The drawing under review shows one solid part. Ordinate dimensions are in mm from its lowest x, y, z. Round coordinates to 2 decimals unless told otherwise and drop trailing zeros. Write each loop counter-clockwise with the first axis right and the second up, starting at its lowest first coordinate (ties: lowest second). Pieces come first, ordered by that corner, then holes. Notation, with made-up numbers: (50.5, 43) -> (64.5, 43) arc R20 cw to (64.5, 65) -> close; hole circle Ø8 at (16.5, -20.5). An arc over 180 degrees is marked (long way). Use CSV: the item, a comma, the result in double quotes. Start each with the question number.
1) Take a section at D-D, the plane z = 1.5. Give the boundary of the cut face in (x, y), then the cut area to 3 significant figures.
2) Wall thickness on probe 1 along X at (y, z) = (19.8, 1.2) (1 decimal); probe 2 along Z at (x, y) = (33.5, 18.5); probe 3 along Y at (x, z) = (21, 1.25): over which ranges is each line inside the solid? List them lowest first. Write a range as [from, to].
3) Take a section at B-B, the plane z = 5.5. Give the boundary of the cut face in (x, y).
4) For pin 1 Ø4 at (x, y) = (9.5, 19.8) entering from -Z; pin 2 Ø4 at (x, y) = (32.75, 6.38) entering from +Z, all flat-tipped, find the tip position at first contact; note any pin that passes through.
5) Take a section at A-A, the plane x = 25. Give the boundary of the cut face in (y, z).
6) Mouldability with a two-part tool opening along X and no side actions: class the marked faces 1, 2 and 3 as released by +X, released by -X, zero draft, split by the parting line, or undercut.
7) Take a section at C-C, the plane y = 19.8. Give the boundary of the cut face in (x, z).
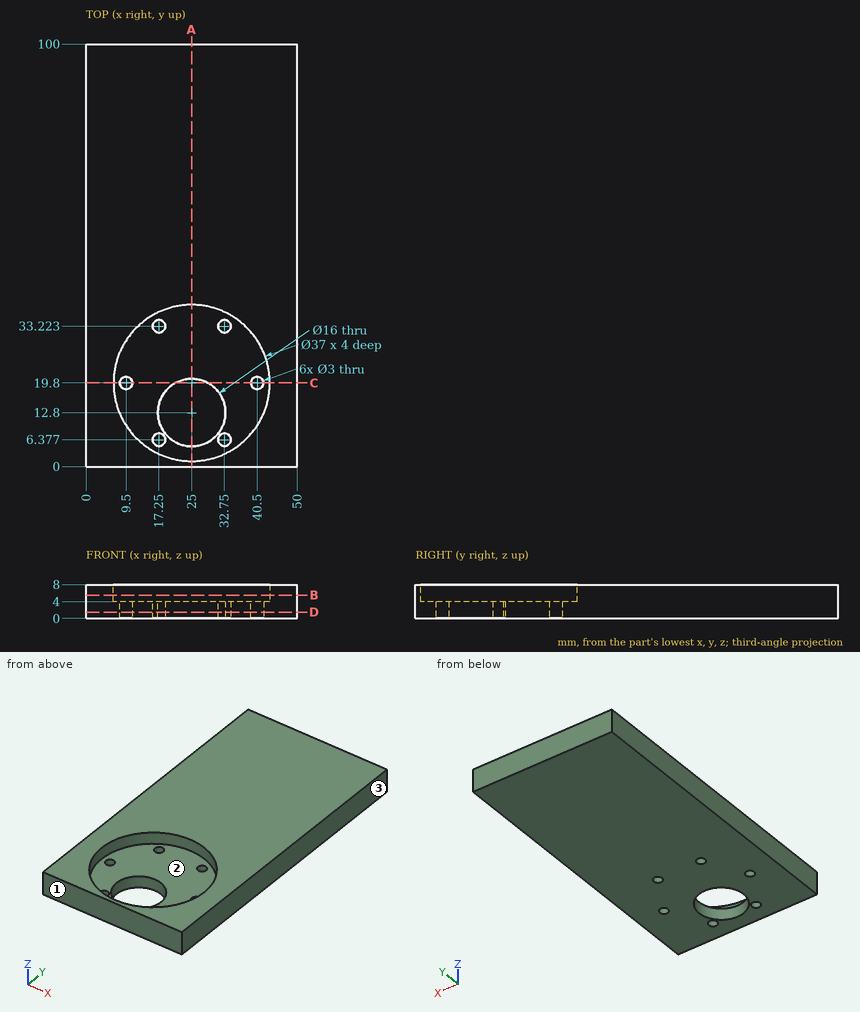
Values found:
1,outline,"(0, 0) -> (50, 0) -> (50, 100) -> (0, 100) -> close; hole circle Ø3 at (9.5, 19.8); hole circle Ø3 at (17.25, 6.38); hole circle Ø3 at (17.25, 33.22); hole circle Ø16 at (25, 12.8); hole circle Ø3 at (32.75, 6.38); hole circle Ø3 at (32.75, 33.22); hole circle Ø3 at (40.5, 19.8)"
1,area,"4,760 mm²"
2,probe 1,"[0, 8], [11, 21.1], [28.9, 39], [42, 50]"
2,probe 2,"[0, 4]"
2,probe 3,"[0, 5.87], [19.73, 100]"
3,outline,"(0, 0) -> (50, 0) -> (50, 100) -> (0, 100) -> close; hole circle Ø37 at (25, 19.8)"
4,pin 1,"z = 0"
4,pin 2,"z = 4"
5,outline,"(0, 0) -> (4.8, 0) -> (4.8, 4) -> (1.3, 4) -> (1.3, 8) -> (0, 8) -> close; (20.8, 0) -> (100, 0) -> (100, 8) -> (38.3, 8) -> (38.3, 4) -> (20.8, 4) -> close"
6,face 1,"zero draft"
6,face 2,"undercut"
6,face 3,"released by +X"
7,outline,"(0, 0) -> (8, 0) -> (8, 4) -> (6.5, 4) -> (6.5, 8) -> (0, 8) -> close; (11, 0) -> (21.13, 0) -> (21.13, 4) -> (11, 4) -> close; (28.87, 0) -> (39, 0) -> (39, 4) -> (28.87, 4) -> close; (42, 0) -> (50, 0) -> (50, 8) -> (43.5, 8) -> (43.5, 4) -> (42, 4) -> close"
